Can you work these out from the model? Positions are in its coordinate system, mm. A direction names the side the tool comes from. Coordinates: 2 decimals unless noted, no trailing zeros. Order: outer loops, then holes, each group sorted by start corner. A loop starts at its lowest first (then second) coordinate and runs counter-clockwise, first axis right, second up.
Autodesk Inventor part; units mm, degrees
ref_plane "YZ Plane" through (0, 0, 0) normal (1, 0, 0) x (0, 1, 0)
ref_plane "XZ Plane" through (0, 0, 0) normal (0, 1, 0) x (-1, 0, 0)
ref_plane "XY Plane" through (0, 0, 0) normal (0, 0, 1) x (1, 0, 0)
sketch "스케치1" plane through (0, 0, 0) normal (0, 1, 0) x (-1, 0, 0)
  line L0 (-2.4, 4.8) -> (2.4, 4.8)
  line L1 (2.4, 4.8) -> (2.4, -4.8)
  line L2 (2.4, -4.8) -> (-2.4, -4.8)
  line L3 (-2.4, -4.8) -> (-2.4, 4.8)
  line L4 (-2.4, 4.8) -> (2.4, -4.8) construction
  line L5 (2.4, 4.8) -> (-2.4, -4.8) construction
  circle A0 centre (0, 0) radius 2.7
  circle A1 centre (0, 0) radius 1.7
  dimension "d0" = 4.8
  dimension "d1" = 9.6
  dimension "d17" = 5.4
  dimension "d18" = 3.4
extrude "돌출1" add sketch "스케치1" along normal blind 0.6 contours L0 L1 A0 L3 | A0 L1 L3 | A0 L1 L2 L3 | A1
sketch "스케치2" plane through (0, 0, 0) normal (0, -1, 0) x (1, 0, 0)
  line L0 (2.4, -4.8) -> (-2.4, -4.8)
  line L1 (2.4, 4.8) -> (2.4, -4.8)
  line L2 (-2.4, 4.8) -> (2.4, 4.8)
  line L3 (-2.4, -4.8) -> (-2.4, 4.8)
  line L4 (2.4, 4.8) -> (3, 4.8)
  line L5 (3, 4.8) -> (3, -4.8)
  line L6 (3, -4.8) -> (2.4, -4.8)
  line L7 (2.4, -4.8) -> (2.4, 4.8)
  line L8 (-2.4, -4.8) -> (-2.4, 4.8)
  line L9 (-2.4, 4.8) -> (-3, 4.8)
  line L10 (-3, 4.8) -> (-3, -4.8)
  line L11 (-3, -4.8) -> (-2.4, -4.8)
  line L12 (-2.4, -4.8) -> (-2.4, 4.8)
  point P0 (0, 0)
  dimension "d4" = 0.6
  dimension "d5" = 0.6
extrude "돌출2" add sketch "스케치2" against normal blind 3.1 contours L1 L4 L5 L6 | L11 L10 L9 L3
extrude "돌출5" add sketch "스케치1" against normal blind 2.5 contours A0 L1 L3 | L3 A0 | A0 L1
properties part number "endcap_4mm_2ea_typeB_ver2_onyx_addon"
1. Imagine slicing it at B-B on z = 0. Please give me the cut outline in (x, y).
Completed:
outline: (-3, 0) - (-2.7, 0) - (-2.7, -2.5) - (-1.7, -2.5) - (-1.7, 0) - (1.7, 0) - (1.7, -2.5) - (2.7, -2.5) - (2.7, 0) - (3, 0) - (3, 3.1) - (2.4, 3.1) - (2.4, 0.6) - (-2.4, 0.6) - (-2.4, 3.1) - (-3, 3.1) - close
2. Imagine slicing it at A-A on y = 2.7. Please give me the cut outline in (x, z), then the cut area to 3 significant figures.
Completed:
outline: (-3, -4.8) - (-2.4, -4.8) - (-2.4, 4.8) - (-3, 4.8) - close; (2.4, -4.8) - (3, -4.8) - (3, 4.8) - (2.4, 4.8) - close
area: 11.5 mm2
3. Please list where these lines run through material, in increasing order: probe 1 along X at (y, z) = (0.85, -3.5); probe 2 along Z at (x, y) = (0, -1.45); probe 3 along Y at (x, z) = (1.3, -1).
Completed:
probe 1: x = -3 to -2.4, 2.4 to 3
probe 2: z = -2.7 to -1.7, 1.7 to 2.7
probe 3: y = 0 to 0.6
4. Imagine slicing it at C-C on x = -2. Please give me the cut outline in (y, z), then the cut area to 3 significant figures.
Completed:
outline: (-2.5, -1.81) - (0, -1.81) - (0, -4.8) - (0.6, -4.8) - (0.6, 4.8) - (0, 4.8) - (0, 1.81) - (-2.5, 1.81) - close
area: 14.8 mm2
5. On a 3-axis mill with a long thin cutter (end or side, diameter ignored), from which of +Z, -Z, +X, -X, +Y, -Y can I reach the whole of each face in a straight line? I mean faces 4 (the flat face through (0, -2.5, -2)), 5 (the flat face through (-2.4, 2, 0)), 6 (the flat face through (0, 0, 0)). Say none if no direction works.
Completed:
face 4: +Z, -Z, +X, -X, -Y
face 5: +Z, -Z, +Y
face 6: -Y
6. Imagine slicing it at D-D on y = -0.6. Please give me the cut outline in (x, z).
Completed:
outline: circle Ø5.4 at (0, 0); hole circle Ø3.4 at (0, 0)
7. Thinking about a two-plate mould opening in X: for faces 1 (the flat face through (0, 0.6, 0)), 2 (the flat face through (-3, 2, 0)), 3 (the flat face through (0, 0.2, -4.8)), which applies, pulls with the +X half, pulls with the -X half, needs draft (parallel to the pull), parting line crosses it, or undercut?
Completed:
face 1: undercut
face 2: pulls with the -X half
face 3: needs draft
8. I'm going to push flat-ended pins straight in: pin 1 (2 mm diameter, centred on x = 0, z = 0, fed in from -Y); pin 2 (1.4 mm diameter, centred on x = -0.5, z = -0.5, fed in from +Y); pin 3 (3 mm diameter, centred on x = -1, z = -0.5, fed in from -Y). Where does each tip first touch, or does it pass through?
Completed:
pin 1: stops at y = 0
pin 2: stops at y = 0.6
pin 3: stops at y = -2.5
